from build123d import *

# Parameters (mm, degrees)
F1_DEPTH = 7.112
F2_R     = 2.54
F3_R     = 2.54


with BuildPart() as f1:
    # F0 (on Front) → F1 (new body)
    with BuildSketch(Plane.XZ):
        Polygon((-28.863836, -17.969469), (-9.111056, -17.969469), (-9.385372, -12.106972), (-22.452589, -12.106972), (-22.452589, 2.791757), (-28.863836, 2.791757), align=None)
    extrude(amount=F1_DEPTH)

    # F2
    f2_edges = [f1.edges().sort_by_distance(p)[0] for p in [
        (-28.863836, -7.112, -7.588856),
    ]]
    fillet(f2_edges, radius=F2_R)

    # F3
    f3_edges = [f1.edges().sort_by_distance(p)[0] for p in [
        (-28.863836, 0, -7.588856),
        (-18.987446, 0, -17.969469),
        (-17.717446, -7.112, -17.969469),
    ]]
    fillet(f3_edges, radius=F3_R)


solid = f1.part
Design review of the part built by this model. Coordinates are the model's own, in mm. A direction names the side the tool comes from. Round coordinates to 2 decimals unless told otherwise and drop trailing zeros. Loops run counter-clockwise (first coordinate to the right, second up) from the corner with the lowest first, then second, coordinate; pieces in that order, holes last. Notation, with made-up numbers: (61.25, 32.5) - (68.25, 32.5) arc R25 ccw to (68.25, 53.5) - close; hole circle Ø5 at (84.25, 18.5). An arc over 180 degrees is marked (long way). One line per item, written item: value. Start each with the question number.
1) To check wall thickness, follow L1, parallel to Z at x = -16.25, y = -3.25; L2, parallel to Z at x = -26.5, y = -3.5; L3, parallel to X at y = -4.5, z = -3.75. State the ranges of each line that lie inside material, in increasing order. Write a range as from..to.
2) Insertion check: pin 1 Ø3 at (x, y) = (-23, -6.5) entering from -Z. The pin has a flat end and moves straight along its axis. Give the tip position at first contact, or say it passes through.
3) Consider section D-D on y = -0.5. Give the boundary of the cut face in (x, z), then the cut area to 3 significant figures.
4) Consider section B-B on x = -20. Give the boundary of the cut face in (y, z), then the cut area to 3 significant figures.
5) Consider section A-A on y = -3.5. Give the boundary of the cut face in (x, z), then the cut area to 3 significant figures.
6) Consider section C-C on z = -8. Give the boundary of the cut face in (x, y).
7) For faces 1 (the flat face through (-16, -4, -12.107)), 2 (the flat face through (-24, 0, -10)), list the 3-axis set-ups (+Z, -Z, +X, -X, +Y, -Y) from which the entire face can be reached by the end or side of a thin tool; tool diameter is ignored.
Reported:
1. L1: z = -17.97..-12.11
1. L2: z = -17.96..2.79
1. L3: x = -28.86..-22.45
2. pin 1: stops at z = -17.93
3. outline: (-27.84, -15.43) arc R1.51 ccw to (-26.32, -16.94) - (-9.16, -16.94) - (-9.39, -12.11) - (-22.45, -12.11) - (-22.45, 2.79) - (-27.84, 2.79) - close
3. area: 170 mm^2
4. outline: (-7.11, -15.43) arc R2.54 ccw to (-4.57, -17.97) - (-2.54, -17.97) arc R2.54 ccw to (0, -15.43) - (0, -12.11) - (-7.11, -12.11) - close
4. area: 38.9 mm^2
5. outline: (-28.86, -15.43) arc R2.54 ccw to (-26.32, -17.97) - (-9.11, -17.97) - (-9.39, -12.11) - (-22.45, -12.11) - (-22.45, 2.79) - (-28.86, 2.79) - close
5. area: 209 mm^2
6. outline: (-28.86, -4.57) arc R2.54 ccw to (-26.32, -7.11) - (-22.45, -7.11) - (-22.45, 0) - (-26.32, 0) arc R2.54 ccw to (-28.86, -2.54) - close
7. face 1: +Z, +X, +Y, -Y
7. face 2: +Z, -Z, +X, -X, +Y
